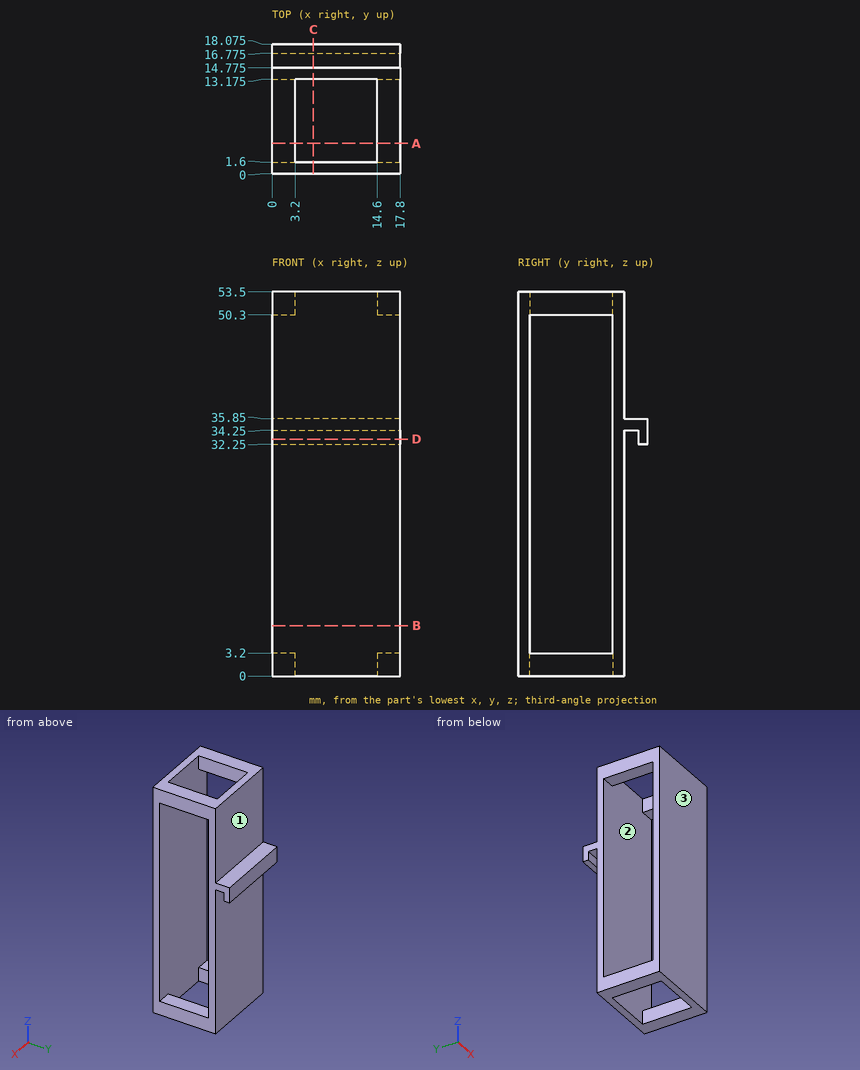
Geometry check sheet. Reference: drawing and pictorial views, mm from the part's lowest x, y, z. Coordinates: 2 decimals unless noted, no trailing zeros. Write each loop counter-clockwise with the first axis right and the second up, starting at its lowest first coordinate (ties: lowest second). Pieces come first, ordered by that corner, then holes. Notation, with made-up numbers: (-18, -11.5) - (12, -11.5) arc R26 ccw to (12, 20.5) - close; hole circle Ø2 at (4.5, 26.5). An arc over 180 degrees is marked (long way). One line per question, with ' | ' between items. Start each with the question number.
1. Gauge pin test, flat ends, axial feed: P1, Ø3.5, axis at x = 9, y = 17, coming from the +Z side; P2, Ø0.6, axis at x = 9.5, y = 15.5, coming from the -Z side; P3, Ø1, axis at x = 10.5, y = 17.5, coming from the -Z side. Record the tip position at first contact, or that the pin passes through.
2. Material ranges on line 1 along Z through (x, y) = (2.75, 5.5); line 2 along Y through (x, z) = (7.75, 43) (3 decimals); line 3 along Y through (x, z) = (7, 33.5) (3 decimals), recorded low to high.
3. Draft check along Y on the marked faces 1, 2 and 3. Enter one of: released by +Y, released by -Y, zero draft, split by the parting line, or undercut.
4. Section check C-C (x = 5.75). Enter the section's corners in (y, z) (3 decimals).
5. Section check B-B (z = 7). Enter the section's corners in (x, y) (3 decimals), plus the area to 3 significant figures.
6. Section check A-A (y = 4.25). Enter the section's corners in (x, z).
7. Section check D-D (z = 33). Enter the section's corners in (x, y) (3 decimals), plus the area to 3 significant figures.
Computed values:
1) P1: z = 35.85 | P2: z = 34.25 | P3: z = 32.25
2) line 1: 0 to 3.2, 50.3 to 53.5 | line 2: 0 to 1.6, 13.175 to 14.775 | line 3: 0 to 1.6, 13.175 to 14.775, 16.775 to 18.075
3) face 1: released by +Y | face 2: undercut | face 3: released by -Y
4) outline: (0, 0) - (1.6, 0) - (1.6, 53.5) - (0, 53.5) - close; (13.175, 0) - (14.775, 0) - (14.775, 34.25) - (16.775, 34.25) - (16.775, 32.25) - (18.075, 32.25) - (18.075, 35.85) - (14.775, 35.85) - (14.775, 53.5) - (13.175, 53.5) - close
5) outline: (0, 0) - (17.8, 0) - (17.8, 1.6) - (0, 1.6) - close; (0, 13.175) - (17.8, 13.175) - (17.8, 14.775) - (0, 14.775) - close | area: 57.0 mm²
6) outline: (0, 0) - (3.2, 0) - (3.2, 3.2) - (0, 3.2) - close; (0, 50.3) - (3.2, 50.3) - (3.2, 53.5) - (0, 53.5) - close; (14.6, 0) - (17.8, 0) - (17.8, 3.2) - (14.6, 3.2) - close; (14.6, 50.3) - (17.8, 50.3) - (17.8, 53.5) - (14.6, 53.5) - close
7) outline: (0, 0) - (17.8, 0) - (17.8, 1.6) - (0, 1.6) - close; (0, 13.175) - (17.8, 13.175) - (17.8, 14.775) - (0, 14.775) - close; (0, 16.775) - (17.8, 16.775) - (17.8, 18.075) - (0, 18.075) - close | area: 80.1 mm²
